from build123d import *

# Parameters (mm, degrees)
F0_W     = 16
F0_H     = 8
F0_W_2   = 12.8
F0_H_2   = 4.8
F1_DEPTH = 9.6
F2_DEPTH = 8
F3_R     = 1.6
F4_DEPTH = 1.6
F5_R     = 2.4
F6_DEPTH = 1.6


with BuildPart() as f1:
    # F0 (on Top) → F1 (new body)
    with BuildSketch(Plane.XY):
        Rectangle(F0_W, F0_H)
        Rectangle(F0_W_2, F0_H_2, mode=Mode.SUBTRACT)
        Rectangle(F0_W_2, F0_H_2)
    extrude(amount=F1_DEPTH)

    # F0 (on Top) → F2 (cut)
    with BuildSketch(Plane.XY):
        Rectangle(F0_W_2, F0_H_2)
    extrude(amount=F2_DEPTH, mode=Mode.SUBTRACT)

    # F3 (on face) → F4 (cut)
    with BuildSketch(Plane.XY.offset(9.6)):
        with Locations((4, 0)):
            Circle(F3_R)
        with Locations((-4, 0)):
            Circle(F3_R)
    extrude(amount=-F4_DEPTH, mode=Mode.SUBTRACT)

    # F5 (on face) → F6 (join)
    with BuildSketch(Plane.XY.offset(9.6)):
        with Locations((-4, 0)):
            Circle(F5_R)
        with Locations((4, 0)):
            Circle(F5_R)
    extrude(amount=F6_DEPTH)


solid = f1.part
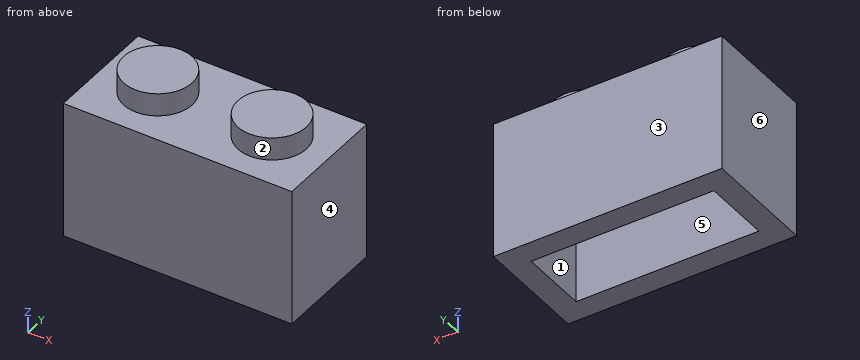
The model under review builds one solid part; all positions refer to its coordinate system, in mm. Face numbers are marked on the shaded views. A direction names the side the tool comes from. Give positions to 0.01 mm unless a question says otherwise; leave off trailing zeros. Order: outer loops, then holes, each group sorted by start corner. A loop starts at its lowest first (then second) coordinate and runs counter-clockwise, first axis right, second up. Notation, with made-up numbers: M 81,26 L 123,26 A14 cw 123,53 Z; hole C -10.5,-35.5 d3. An arc over 180 degrees is marked long. One line per question, with ' | ' between items. Start each with the question number.
1) For the marked faces 1, 2 and 3, list the 3-axis set-ups (+Z, -Z, +X, -X, +Y, -Y) from which the entire face can be reached by the end or side of a thin tool; tool diameter is ignored.
2) Wall thickness on L1, parallel to X at y = 1.25, z = 6.25; L2, parallel to Y at x = 3.25, z = 4.75; L3, parallel to Y at x = -4, z = 8.55: over which ranges is each line inside the solid? List them lowest first. Write a range as from..to.
3) Consider section B-B, the plane y = 0. Give the boundary of the cut face in (x, z).
4) Consider section C-C, the plane x = -4. Give the boundary of the cut face in (y, z).
5) Consider section A-A, the plane z = 7. Give the boundary of the cut face in (x, y), then the cut area to 3 significant figures.
6) Mouldability with a two-part tool opening along X and no side actions: class the marked faces 4, 5 and 6 as pulls with the +X half, pulls with the -X half, needs draft (parallel to the pull), parting line crosses it, or undercut.
7) Clearance check with flat-ended pins moving along their axes: P1, Ø3.5, axis at x = 4.5, y = 0, coming from the -Z side; P2, Ø1.5, axis at x = -1.5, y = 2, coming from the +Z side. State where each tip first meets the part, or that it passes through.
8) Consider section D-D, the plane x = -0.75. Give the boundary of the cut face in (y, z), then the cut area to 3 significant figures.
Found:
1) face 1: -Z | face 2: +Z | face 3: +Z, -Z, +X, -X, +Y
2) L1: x = -8..-6.4, 6.4..8 | L2: y = -4..-2.4, 2.4..4 | L3: y = -4..-1.6, 1.6..4
3) outline: M -8,0 L -6.4,0 L -6.4,8 L -5.6,8 L -5.6,9.6 L -2.4,9.6 L -2.4,8 L 2.4,8 L 2.4,9.6 L 5.6,9.6 L 5.6,8 L 6.4,8 L 6.4,0 L 8,0 L 8,9.6 L 6.4,9.6 L 6.4,11.2 L 1.6,11.2 L 1.6,9.6 L -1.6,9.6 L -1.6,11.2 L -6.4,11.2 L -6.4,9.6 L -8,9.6 Z
4) outline: M -4,0 L -2.4,0 L -2.4,8 L -1.6,8 L -1.6,9.6 L 1.6,9.6 L 1.6,8 L 2.4,8 L 2.4,0 L 4,0 L 4,9.6 L 2.4,9.6 L 2.4,11.2 L -2.4,11.2 L -2.4,9.6 L -4,9.6 Z
5) outline: M -8,-4 L 8,-4 L 8,4 L -8,4 Z; hole M -6.4,-2.4 L 6.4,-2.4 L 6.4,2.4 L -6.4,2.4 Z | area: 66.6 mm²
6) face 4: pulls with the +X half | face 5: undercut | face 6: pulls with the -X half
7) P1: stops at z = 8 | P2: stops at z = 9.6
8) outline: M -4,0 L -2.4,0 L -2.4,8 L 2.4,8 L 2.4,0 L 4,0 L 4,9.6 L -4,9.6 Z | area: 38.4 mm²
